Could you check a few things on this drawing? It's one solid part, dimensions in mm from its lowest x, y, z. Give positions to 0.01 mm unless a question says otherwise; leave off trailing zeros. Order: outer loops, then holes, each group sorted by start corner. A loop starts at its lowest first (then second) coordinate and runs counter-clockwise, first axis right, second up. Notation, with made-up numbers: M 47.25,12.25 L 105.25,12.25 A17 cw 105.25,27.25 Z; hole C 88.25,9.5 d4. An arc over 180 degrees is marked long. Use one line per item in the form item = value. Start each with the question number.
1. I want a section at A-A, the plane y = 0.9. List the corners of the cut face in (x, z) for me.
2. I want a section at B-B, the plane z = 6. List the corners of the cut face in (x, y) for me.
3. I want a section at C-C, the plane x = 14. List the corners of the cut face in (y, z) for me, and give its area (3 significant figures).
4. I need wall thicknesses on L1, parallel to Y at x = 18.3, z = 2; L2, parallel to Z at x = 1.75, y = 2.65; L3, parallel to X at y = 2.4, z = 5. Which ranges of each line are inside material? Lowest first, please.
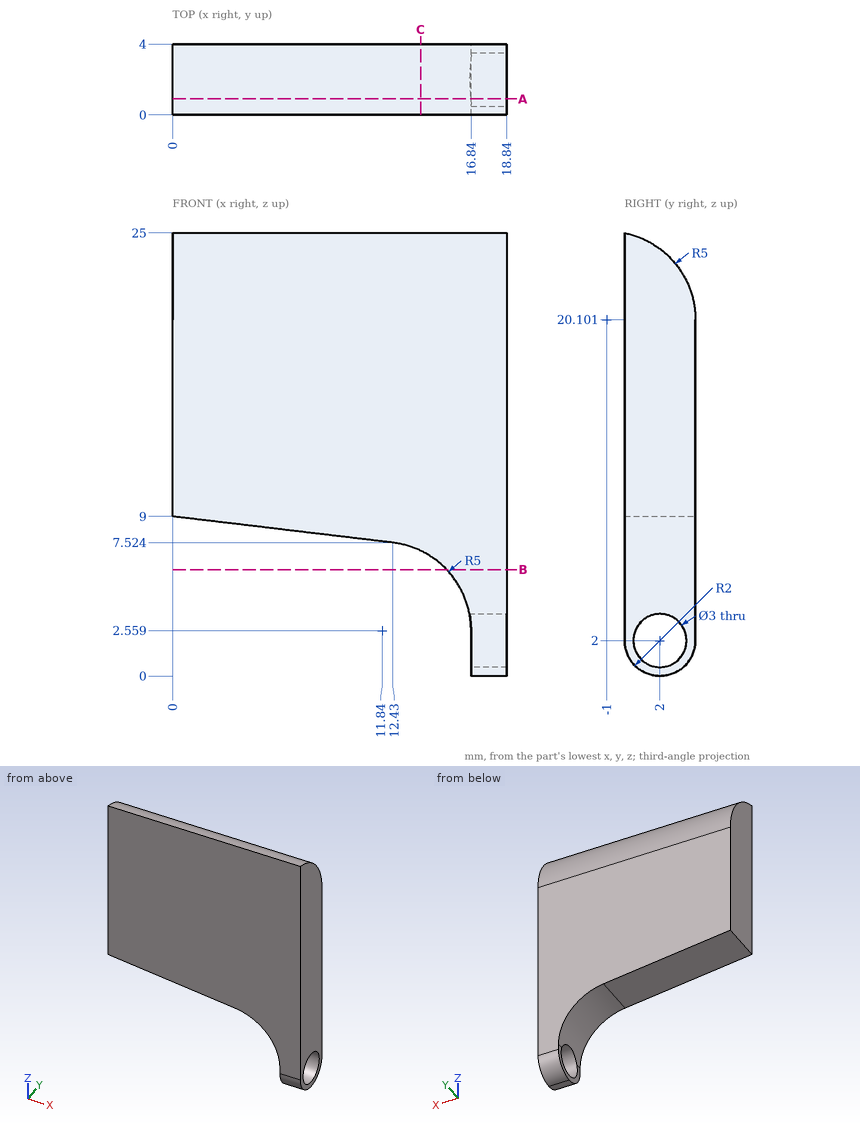
Check result:
q1.outline = M 0,9 L 12.43,7.52 A5 cw 16.82,3.02 L 18.84,3.02 L 18.84,24.73 L 0,24.73 Z; M 16.84,0.33 L 18.84,0.33 L 18.84,0.98 L 16.84,0.98 Z
q2.outline = M 15.47,0 L 18.84,0 L 18.84,4 L 15.47,4 Z
q3.outline = M 0,7.07 L 4,7.07 L 4,20.1 A5 ccw 0,25 Z
q3.area = 66.8 mm2
q4.L1 = 0 to 0.5, 3.5 to 4
q4.L2 = 8.79 to 23.52
q4.L3 = 16.2 to 18.84
